Study the drawing (mm; zero at the part's minimum x, y, z) and answer. A direction names the side the tool comes from. Round coordinates to 2 decimals unless told otherwise and drop trailing zeros. Write each loop counter-clockwise with the first axis right and the second up, starting at its lowest first coordinate (ties: lowest second). Pieces come first, ordered by that corner, then holes.
(1) A cutting plane is placed at C-C, the plane x = 15.75. Give the vertices of the cut face in (y, z).
(2) A cutting plane is placed at A-A, the plane x = 6. Give the vertices of the cut face in (y, z).
(3) Find the intervals of material crossed by probe 1 along Z at (x, y) = (17.5, 6); probe 2 along Y at (x, z) = (10, 23.85); probe 3 along Z at (x, y) = (13.25, 6), in increasing order.
(4) The mould has two halves that part along Z. Classify the marked faces 1, 2, 3 and 4: +Z half, -Z half, draft (parallel to the pull), parting line (faces both ways), or undercut.
(5) Each of these flat-tipped pins is pushed along its axis until it touches: pin 1 Ø1.1 at (x, z) = (12, 3.5) entering from +Y; pin 2 Ø3 at (x, y) = (9, 4) entering from -Z; pin 3 Ø4.5 at (x, y) = (25, 5) entering from -Z; pin 4 Ø1.9 at (x, z) = (6, 15.5) entering from -Y. Where does it stop, or does it pass through?
(6) For the marked faces 5, 6, 7 and 8, determine the directions among +Z, -Z, +X, -X, +Y, -Y from which every point of the face is accessible in a straight line to the end or side of a thin tool.
(7) A cutting plane is placed at D-D, the plane z = 6. Give the vertices of the cut face in (x, y).
(8) A cutting plane is placed at B-B, the plane y = 6. Give the number of separate pieces and of enclosed holes in the cut face, and give its area (3 significant figures).
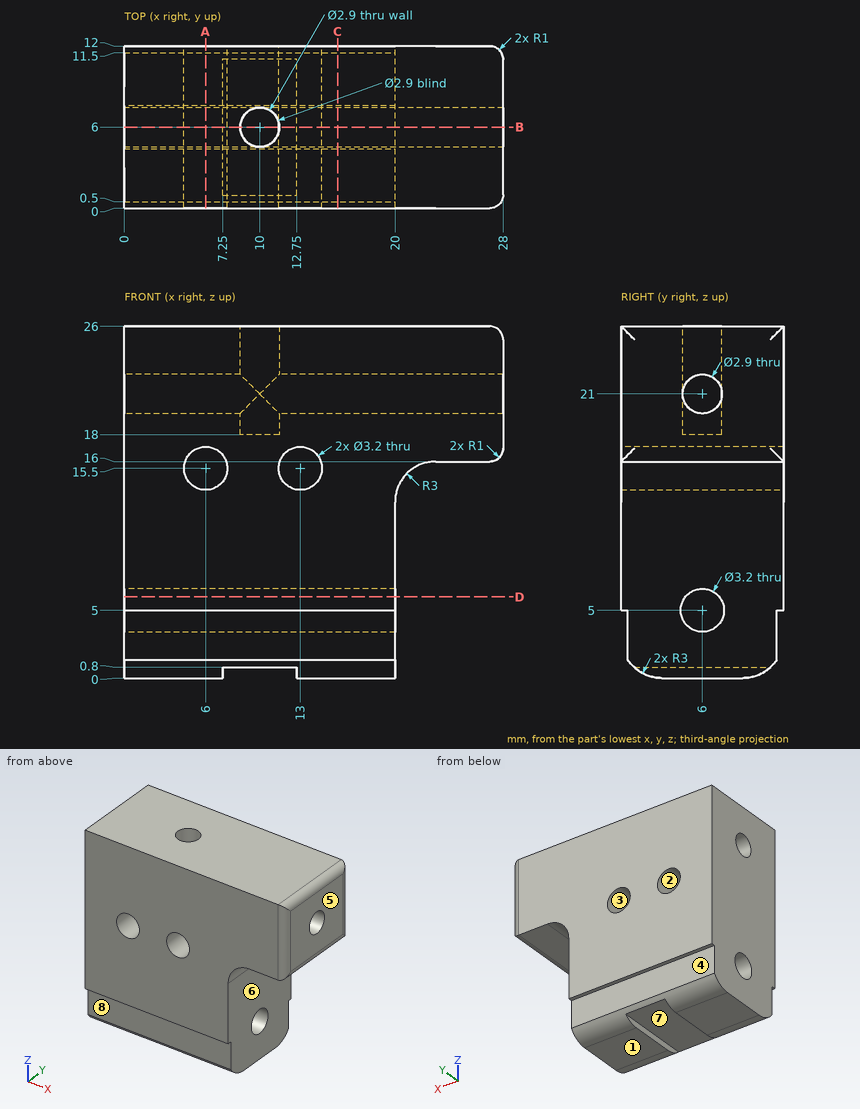
Solutions:
1. outline: (0, 5) - (0.5, 5) - (0.5, 1.34) arc R3 ccw to (3, 0) - (9, 0) arc R3 ccw to (11.5, 1.34) - (11.5, 5) - (12, 5) - (12, 26) - (0, 26) - close; hole circle Ø3.2 at (6, 5); hole circle Ø2.9 at (6, 21)
2. outline: (0, 5) - (0.5, 5) - (0.5, 1.34) arc R3 ccw to (3, 0) - (9, 0) arc R3 ccw to (11.5, 1.34) - (11.5, 5) - (12, 5) - (12, 13.9) - (0, 13.9) - close; (0, 17.1) - (12, 17.1) - (12, 26) - (0, 26) - close; hole circle Ø3.2 at (6, 5); hole circle Ø2.9 at (6, 21)
3. probe 1: z = 0 to 3.4, 6.6 to 19.55, 22.45 to 26
3. probe 2: y = 0 to 4.55, 7.45 to 12
3. probe 3: z = 0 to 3.4, 6.6 to 13.92, 17.08 to 19.55, 22.45 to 26
4. face 1: -Z half
4. face 2: undercut
4. face 3: undercut
4. face 4: draft
5. pin 1: stops at y = 11.5
5. pin 2: stops at z = 0.8
5. pin 3: stops at z = 15.99
5. pin 4: passes through
6. face 5: +Z, -Z, +X, +Y, -Y
6. face 6: -Z, +X, +Y, -Y
6. face 7: -Z, +Y, -Y
6. face 8: -Z, +X, -X, -Y
7. outline: (0, 0) - (20, 0) - (20, 4.75) - (0, 4.75) - close; (0, 7.25) - (20, 7.25) - (20, 12) - (0, 12) - close
8. separate pieces: 4
8. enclosed holes: 2
8. area: 421 mm2
